Design review of the part built by this model. Coordinates are the model's own, in mm. Face numbers are marked on the shaded views. Coordinates: 2 decimals unless noted, no trailing zeros. Loops run counter-clockwise (first coordinate to the right, second up) from the corner with the lowest first, then second, coordinate; pieces in that order, holes last. Notation, with made-up numbers: M 41.25,5 L 84.25,5 A20 ccw 84.25,14 Z; hole C 36,38 d2. An arc over 180 degrees is marked long. Put each result on its own line as item: value. Start each with the question number.
(1) The part is to be moulded in two halves that separate along Y. For the marked faces 1, 2 and 3, say which applies: +Y half, -Y half, draft (parallel to the pull), parting line (faces both ways), or undercut.
(2) Take a section at A-A, the plane y = 0. Give the boundary of the cut face in (x, z), then the cut area to 3 significant figures.
(3) Take a section at B-B, the plane x = 0. Give the boundary of the cut face in (y, z), then the cut area to 3 significant figures.
(4) Take a section at C-C, the plane z = 20.5. Give the boundary of the cut face in (x, y), then the cut area to 3 significant figures.
(5) For probe 1 along Y at (x, z) = (0, 10); probe 2 along Y at (x, z) = (-9, 6.5); probe 3 along X at (y, z) = (12, 9), list the stretches that pass through material, from the lowest coordinate up. Write a range as [from, to].
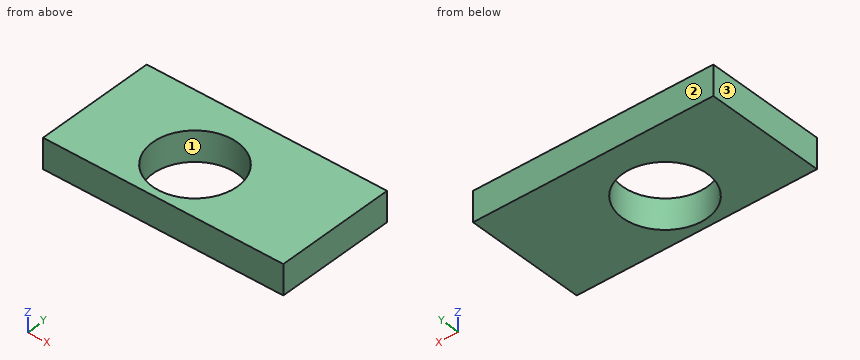
```python
from build123d import *

# Parameters (mm, degrees)
F0_W     = 200
F0_H     = 100
F0_R     = 35.191304
F1_DEPTH = 25
F3_W     = 11.49768
F3_H     = 100
F4_DEPTH = 10
F5_W     = 11.49768
F5_H     = 100
F6_DEPTH = 10


with BuildPart() as f1:
    # F0 (on Top) → F1 (new body)
    with BuildSketch(Plane.XY):
        with Locations((9.423193, 8.395134)):
            Rectangle(F0_W, F0_H)
        Circle(F0_R, mode=Mode.SUBTRACT)
    extrude(amount=F1_DEPTH)

    # F3 (on face) → F4 (join)
    with BuildSketch(Plane.XY.offset(25)):
        with Locations((-66.680519, 8.395134)):
            Rectangle(F3_W, F3_H)
    extrude(amount=-F4_DEPTH)

    # F5 (on face) → F6 (join)
    with BuildSketch(Plane.XY.offset(25)):
        with Locations((-66.680519, 8.395134)):
            Rectangle(F5_W, F5_H)
    extrude(amount=-F6_DEPTH)


solid = f1.part
```
Computed values:
1. face 1: undercut
1. face 2: +Y half
1. face 3: draft
2. outline: M -90.58,0 L -35.19,0 L -35.19,25 L -90.58,25 Z; M 35.19,0 L 109.42,0 L 109.42,25 L 35.19,25 Z
2. area: 3,240 mm^2
3. outline: M -41.6,0 L -35.19,0 L -35.19,25 L -41.6,25 Z; M 35.19,0 L 58.4,0 L 58.4,25 L 35.19,25 Z
3. area: 740 mm^2
4. outline: M -90.58,-41.6 L 109.42,-41.6 L 109.42,58.4 L -90.58,58.4 Z; hole C 0,0 d70.38
4. area: 16,100 mm^2
5. probe 1: y = [-41.6, -35.19], [35.19, 58.4]
5. probe 2: y = [-41.6, -34.02], [34.02, 58.4]
5. probe 3: x = [-90.58, -33.08], [33.08, 109.42]
